Autodesk Inventor part; units mm, degrees
ref_plane "YZ Plane" through (0, 0, 0) normal (1, 0, 0) x (0, 1, 0)
ref_plane "XZ Plane" through (0, 0, 0) normal (0, 1, 0) x (-1, 0, 0)
ref_plane "XY Plane" through (0, 0, 0) normal (0, 0, 1) x (1, 0, 0)
sketch "스케치1" plane through (0, 0, 0) normal (0, 0, 1) x (1, 0, 0)
  line L0 (0, 17.4) -> (0, -17.4) construction
  line L1 (-20, 17.4) -> (-20, -17.4)
  line L2 (20, -17.4) -> (20, 17.4)
  arc A0 (20, 17.4) -> (-20, 17.4) centre (0, 17.4) ccw
  arc A1 (-20, -17.4) -> (20, -17.4) centre (0, -17.4) ccw
  point P0 (0, 0)
  point P1 (0, 0)
  dimension "d0" = 34.8
  dimension "d1" = 40
extrude "돌출1" add sketch "스케치1" along normal blind 25
sketch "스케치2" plane through (0, 0, 25) normal (0, 0, 1) x (1, 0, 0)
  circle A0 centre (0, 18.7) radius 18.7
  point P0 (0, 0)
  dimension "d4" = 37.4
extrude "돌출2" add sketch "스케치2" along normal blind 239
sketch "스케치3" plane through (0, 18.7, 264) normal (0, 0, 1) x (1, 0, 0)
  circle A0 centre (0, 0) radius 12.5
  point P0 (0, -18.7)
  dimension "d7" = 25
extrude "돌출3" add sketch "스케치3" along normal blind 34
sketch "스케치5" plane through (0, 0, 0) normal (0, 0, -1) x (-1, 0, 0)
  line L0 (-7.5, 8.75) -> (7.5, 8.75)
  line L1 (7.5, 8.75) -> (7.5, 26.05)
  line L2 (7.5, 26.05) -> (-7.5, 26.05)
  line L3 (-7.5, 26.05) -> (-7.5, 8.75)
  arc A0 (20, 17.4) -> (-20, 17.4) centre (0, 17.4) ccw
  point P0 (0, 0)
  dimension "d10" = 15
  dimension "d11" = 17.3
  dimension "d12" = 8.65
  dimension "d13" = 7.5
extrude "돌출4" add sketch "스케치5" along normal blind 19
sketch "스케치6" plane through (-20, -17.4, 0) normal (-1, 0, 0) x (0, 0, 1)
  circle A0 centre (-10, 34.8) radius 3
  line L0 (-19, 26.15) -> (-19, 43.45)
  line L1 (0, 43.45) -> (-19, 43.45)
  circle A1 centre (289, 34.8) radius 3
  line L2 (0, 0) -> (25, 0)
  point P0 (0, 17.4)
  dimension "d16" = 6
  dimension "d17" = 9
  dimension "d18" = 8.65
  dimension "d19" = 299
  dimension "d20" = 34.8
  dimension "d21" = 6
extrude "돌출5" cut sketch "스케치6" against normal through all
properties part number "높이조절 액추에이터_최대" material "알루미늄 6061"
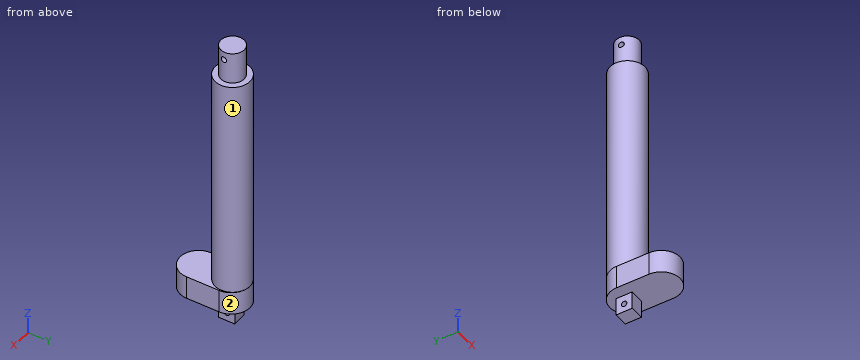
Design review of the part built by this model. Coordinates are the model's own, in mm. Face numbers are marked on the shaded views. A direction names the side the tool comes from. Coordinates: 2 decimals unless noted, no trailing zeros. Order: outer loops, then holes, each group sorted by start corner. A loop starts at its lowest first (then second) coordinate and runs counter-clockwise, first axis right, second up. Notation, with made-up numbers: (35.5, 9) - (59.5, 9) arc R13 ccw to (59.5, 21) - close; hole circle Ø7 at (16.5, -37). An arc over 180 degrees is marked (long way). One line per question, with ' | ' between items.
Q1. For the marked faces 1 and 2, list the 3-axis set-ups (+Z, -Z, +X, -X, +Y, -Y) from which the entire face can be reached by the end or side of a thin tool; tool diameter is ignored.
Answer key:
face 1: +Z | face 2: +Z, -Z, +Y
Q2. Consider section C-C, the plane y = 3. Give the boundary of the cut face in (x, z), then the cut area to 3 significant figures.
Answer key:
outline: (-20, 0) - (20, 0) - (20, 25) - (10.16, 25) - (10.16, 264) - (-10.16, 264) - (-10.16, 25) - (-20, 25) - close | area: 5,860 mm2
Q3. Consider section A-A, the plane z = -10. Give the boundary of the cut face in (x, y), then the cut area to 4 significant figures.
Answer key:
outline: (-7.5, 8.75) - (7.5, 8.75) - (7.5, 14.4) - (-7.5, 14.4) - close; (-7.5, 20.4) - (7.5, 20.4) - (7.5, 26.05) - (-7.5, 26.05) - close | area: 169.5 mm2
Q4. Consider section D-D, the plane z = 270. Give the boundary of the cut face in (x, y).
Answer key:
outline: circle Ø25 at (0, 18.7)
Q5. To check wall thickness, follow line 1 along Z through (x, y) = (0, 17); line 2 along Y through (x, z) = (2, -10); line 3 along X through (y, z) = (33, 14). State the ranges of each line that lie inside material, in increasing order.
Answer key:
line 1: z = -19 to -12.97, -7.03 to 286.03, 291.97 to 298 | line 2: y = 8.75 to 14.4, 20.4 to 26.05 | line 3: x = -12.52 to 12.52
Q6. Consider section B-B, the plane x = -3. Give the number of separate pieces and of enclosed holes in the cut face, then the cut area to 3 significant figures.
Answer key:
separate pieces: 1 | enclosed holes: 2 | area: 11,800 mm2
Q7. Clearance check with flat-ended pins moving along their axes: pin 1 Ø20 at (x, y) = (2, -9.5) entering from -Z; pin 2 Ø9.5 at (y, z) = (17.4, -10) entering from +X; pin 3 Ø14 at (y, z) = (19.5, -9.5) entering from -X; pin 4 Ø5.5 at (y, z) = (17.4, 289) entering from +X. State where each tip first meets the part, or that it passes through.
Answer key:
pin 1: stops at z = 0 | pin 2: stops at x = 7.5 | pin 3: stops at x = -7.5 | pin 4: passes through
